Build history of the part. All positions in model axes, mm. Face numbers are marked on the shaded views. A direction names the side the tool comes from. Coordinates: 2 decimals unless noted, no trailing zeros. Order: outer loops, then holes, each group sorted by start corner. A loop starts at its lowest first (then second) coordinate and runs counter-clockwise, first axis right, second up. Notation, with made-up numbers: (-15, -9) - (4, -9) arc R19 cw to (4, 16) - close; hole circle Ø7 at (16.25, -0.75). An arc over 180 degrees is marked (long way). Write each question's results on one line, items separated by ' | '.
from build123d import *

# Parameters (mm, degrees)
SKETCH_W        = 23.2
SKETCH_H        = 25.8
SKETCH_W_2      = 14.8
SKETCH_H_2      = 16.8
PAD_DEPTH       = 9.75
SKETCH001_W     = 14.8
SKETCH001_H     = 19.8
POCKET_DEPTH    = 8.2
POCKET001_START = -4.2
SKETCH002_W     = 1.5
SKETCH002_H     = 3
POCKET001_DEPTH = 14.8
CHAMFER_SIZE    = 1


with BuildPart() as part:
    # Sketch → Pad (new body)
    with BuildSketch(Plane.XY):
        with Locations((0, 1.5)):
            Rectangle(SKETCH_W, SKETCH_H)
        Rectangle(SKETCH_W_2, SKETCH_H_2, mode=Mode.SUBTRACT)
    extrude(amount=PAD_DEPTH)

    # Sketch001 (on Face10 of Pad) → Pocket (cut)
    with BuildSketch(Plane.XY.offset(9.75)):
        with Locations((0, 1.5)):
            Rectangle(SKETCH001_W, SKETCH001_H)
    extrude(amount=-POCKET_DEPTH, mode=Mode.SUBTRACT)

    # Sketch002 (on Face6 of Pocket) → Pocket001 (cut)
    with BuildSketch(Plane.YZ.offset(11.6).offset(POCKET001_START)):
        with Locations((-9.15, 6.7)):
            Rectangle(SKETCH002_W, SKETCH002_H)
        with Locations((12.15, 6.7)):
            Rectangle(SKETCH002_W, SKETCH002_H)
    extrude(amount=-POCKET001_DEPTH, mode=Mode.SUBTRACT)

    # Chamfer
    chamfer_edges = [part.edges().sort_by_distance(p)[0] for p in [
        (0, 8.4, 1.55),
        (0, 11.4, 9.75),
        (0, -8.4, 9.75),
    ]]
    chamfer(chamfer_edges, length=CHAMFER_SIZE)


solid = part.part
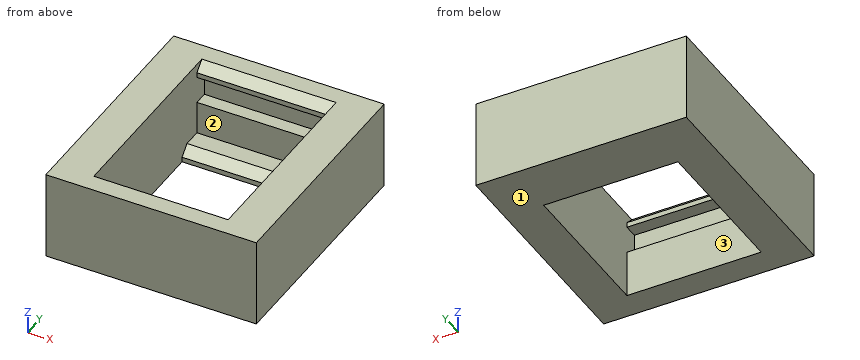
1. Band-saw the part on A-A on y = 2. Give the cut face in (x, z), then the cut area to 3 significant figures.
Solved:
outline: (-11.6, 0) - (-7.4, 0) - (-7.4, 9.75) - (-11.6, 9.75) - close; (7.4, 0) - (11.6, 0) - (11.6, 9.75) - (7.4, 9.75) - close | area: 81.9 mm2
2. Band-saw the part on C-C on z = 6.75. Give the cut face in (x, y), then the cut area to 3 significant figures.
Solved:
outline: (-11.6, -11.4) - (11.6, -11.4) - (11.6, 14.4) - (-11.6, 14.4) - close; hole (-7.4, -9.9) - (7.4, -9.9) - (7.4, 12.9) - (-7.4, 12.9) - close | area: 261 mm2
3. Drop flat-ended pins along their axis: pin 1 Ø0.6 at (x, y) = (0, 11) entering from +Z; pin 2 Ø3 at (x, y) = (-2.5, 6.5) entering from +Z. Give the stop position or say it passes through.
Solved:
pin 1: stops at z = 1.55 | pin 2: passes through
4. Band-saw the part on B-B on x = 3. Give the cut face in (y, z).
Solved:
outline: (-11.4, 0) - (-8.4, 0) - (-8.4, 5.2) - (-9.9, 5.2) - (-9.9, 8.2) - (-8.4, 8.2) - (-8.4, 8.75) - (-9.4, 9.75) - (-11.4, 9.75) - close; (8.4, 0) - (14.4, 0) - (14.4, 9.75) - (12.4, 9.75) - (11.4, 8.75) - (11.4, 8.2) - (12.9, 8.2) - (12.9, 5.2) - (11.4, 5.2) - (11.4, 1.55) - (9.4, 1.55) - (8.4, 0.55) - close
5. Tool access for the marked faces 1, 2 and 3: list every direction of +Z, -Z, +X, -X, +Y, -Y with a clear straight run to the whole face (end or side of a thin tool).
Solved:
face 1: -Z, +X, -X, +Y, -Y | face 2: +Z | face 3: +Z, -Z
6. Probe line 1 (Y direction, x = 3.5, z = 5.25); line 2 (Y direction, x = 4.25, z = 4); line 3 (X direction, y = -5.5, z = 3.75). List the from-to ranges inside material, lowest first.
Solved:
line 1: y = -11.4 to -9.9, 12.9 to 14.4 | line 2: y = -11.4 to -8.4, 11.4 to 14.4 | line 3: x = -11.6 to -7.4, 7.4 to 11.6
7. Band-saw the part on D-D on y = 10.75. Give the cut face in (x, z).
Solved:
outline: (-11.6, 0) - (11.6, 0) - (11.6, 9.75) - (7.4, 9.75) - (7.4, 1.55) - (-7.4, 1.55) - (-7.4, 9.75) - (-11.6, 9.75) - close
